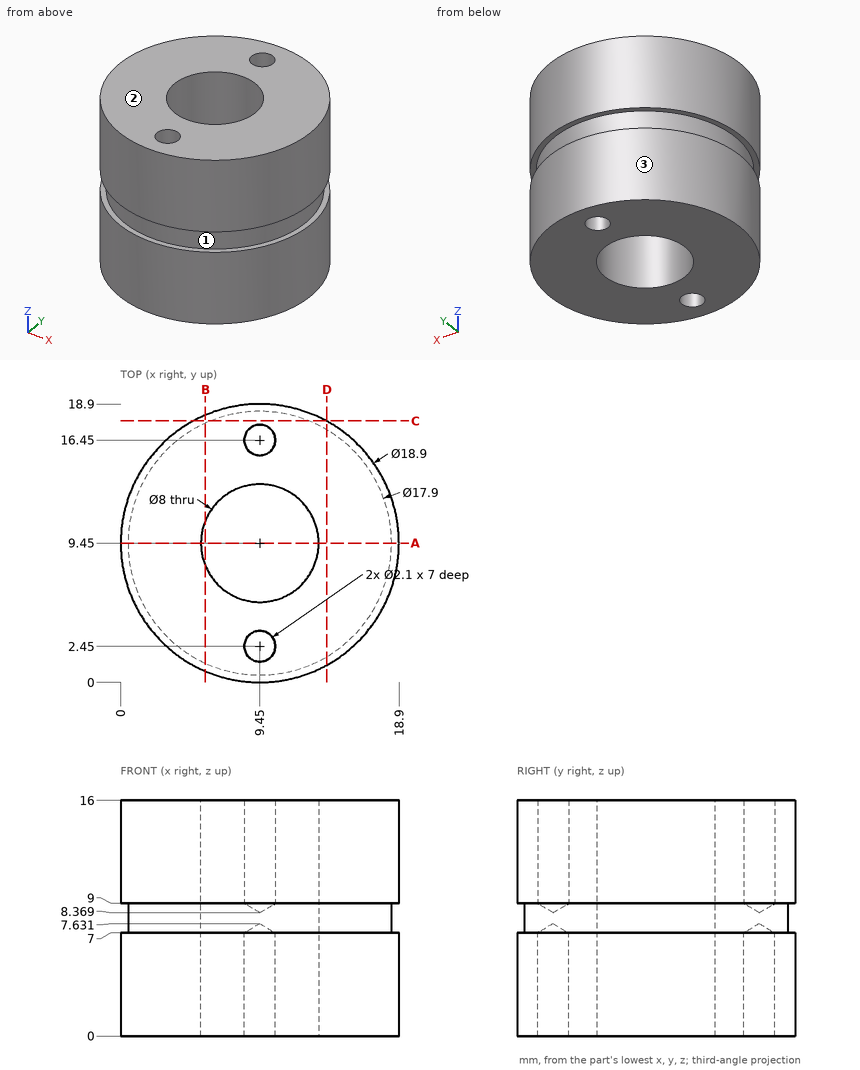
Design review of the part shown in the three views and the two pictorial views. Dimensions are in mm from the part's minimum x, y and z. Give positions to 0.01 mm unless a question says otherwise; leave off trailing zeros. Write each loop counter-clockwise with the first axis right and the second up, starting at its lowest first coordinate (ties: lowest second). Pieces come first, ordered by that corner, then holes. Notation, with made-up numbers: (43.5, 14.5) - (99.5, 14.5) arc R19 ccw to (99.5, 43.5) - close; hole circle Ø2 at (84.5, -24). An arc over 180 degrees is marked (long way). Return JSON: item names as keys, results as strings. Group by question number.
(1) Insertion check: pin 1 (1.5 mm diameter, centred on x = 4, z = 12, fed in from +Y); pin 2 (1.9 mm diameter, centred on x = 9.45, y = 2.45, fed in from -Z); pin 3 (5 mm diameter, centred on x = 15.5, z = 7, fed in from -Y). Each pin has a flat end and moves straight along its axis. Give the tip position at first contact, or say it passes through.
(2) Mouldability with a two-part tool opening along Z and no side actions: class the marked faces 1, 2 and 3 as +Z half, -Z half, draft (parallel to the pull), parting line (faces both ways), or undercut.
(3) To check wall thickness, follow probe 1 along Y at (x, z) = (9.45, 2.5); probe 2 along X at (y, z) = (16.45, 12.5); probe 3 along X at (y, z) = (8.25, 13.75). State the ranges of each line that lie inside material, in increasing order.
(4) We need section B-B, the plane x = 5.75. Give the boundary of the cut face in (y, z).
(5) We need section D-D, the plane x = 14. Give the boundary of the cut face in (y, z).
(6) We need section C-C, the plane y = 17.75. Give the boundary of the cut face in (x, z), then the cut area to 3 significant figures.
(7) We need section A-A, the plane y = 9.45. Give the boundary of the cut face in (x, z).
Reported:
{
 "1": {"pin 1": "stops at y = 17.65", "pin 2": "stops at z = 7.06", "pin 3": "stops at y = 0.69"},
 "2": {"face 1": "undercut", "face 2": "+Z half", "face 3": "draft"},
 "3": {"probe 1": "y = 0 to 1.4, 3.5 to 5.45, 13.45 to 15.4, 17.5 to 18.9", "probe 2": "x = 3.1 to 8.4, 10.5 to 15.8", "probe 3": "x = 0.08 to 5.63, 13.27 to 18.82"},
 "4": {"outline": "(0.75, 0) - (7.93, 0) - (7.93, 16) - (0.75, 16) - (0.75, 9) - (1.3, 9) - (1.3, 7) - (0.75, 7) - close; (10.97, 0) - (18.15, 0) - (18.15, 7) - (17.6, 7) - (17.6, 9) - (18.15, 9) - (18.15, 16) - (10.97, 16) - close"},
 "5": {"outline": "(1.17, 0) - (17.73, 0) - (17.73, 7) - (17.16, 7) - (17.16, 9) - (17.73, 9) - (17.73, 16) - (1.17, 16) - (1.17, 9) - (1.74, 9) - (1.74, 7) - (1.17, 7) - close"},
 "6": {"outline": "(4.93, 0) - (13.97, 0) - (13.97, 7) - (12.8, 7) - (12.8, 9) - (13.97, 9) - (13.97, 16) - (4.93, 16) - (4.93, 9) - (6.1, 9) - (6.1, 7) - (4.93, 7) - close", "area": "140 mm2"},
 "7": {"outline": "(0, 0) - (5.45, 0) - (5.45, 16) - (0, 16) - (0, 9) - (0.5, 9) - (0.5, 7) - (0, 7) - close; (13.45, 0) - (18.9, 0) - (18.9, 7) - (18.4, 7) - (18.4, 9) - (18.9, 9) - (18.9, 16) - (13.45, 16) - close"}
}
